```python
from build123d import *

# Parameters (mm, degrees)
SKETCH1_W               = 50
SKETCH1_H               = 50
SKETCH1_R               = 3.75
SKETCH1_R_2             = 2.75
BOSS_EXTRUDE1_DEPTH     = 3
BOSS_EXTRUDE2_DEPTH     = 50
CUT_EXTRUDE2_DEPTH      = 2
SKETCH10_W              = 50
SKETCH10_H              = 2.047418662
BOSS_EXTRUDE6_DEPTH     = 2
SKETCH11_W              = 5
SKETCH11_H              = 19
CUT_EXTRUDE4_DEPTH      = 4
SKETCH12_W              = 2
SKETCH12_H              = 50
BOSS_EXTRUDE7_DEPTH     = 10
SKETCH13_W              = 19
SKETCH13_H              = 5
CUT_EXTRUDE5_DEPTH      = 10
SKETCH14_R              = 5.75
SKETCH14_R_2            = 3.75
SKETCH14_R_3            = 4.75
SKETCH14_R_4            = 2.75
BOSS_EXTRUDE8_DEPTH     = 5
SKETCH15_W              = 50
SKETCH15_H              = 3
CUT_EXTRUDE6_DEPTH      = 161
CUT_EXTRUDE6_DEPTH_BACK = 15
SKETCH16_R              = 3.75
SKETCH16_R_2            = 2.75
BOSS_EXTRUDE9_DEPTH     = 8
SKETCH17_R              = 3.75
CUT_EXTRUDE7_DEPTH      = 9
SKETCH18_R              = 6
SKETCH18_R_2            = 4.75
BOSS_EXTRUDE10_DEPTH    = 8


with BuildPart() as part:
    # Sketch1 → Boss-Extrude1 (new body)
    with BuildSketch(Plane(origin=(0, 0, 0), x_dir=(1, 0, 0), z_dir=(0, 1, 0))):
        with Locations((0, 8.75)):
            Rectangle(SKETCH1_W, SKETCH1_H)
        Circle(SKETCH1_R, mode=Mode.SUBTRACT)
        with Locations((0, 17.5)):
            Circle(SKETCH1_R_2, mode=Mode.SUBTRACT)
    extrude(amount=BOSS_EXTRUDE1_DEPTH)

    # Sketch2 → Boss-Extrude2 (add)
    with BuildSketch(Plane.XY.offset(16.25)):
        Polygon((-25, 0), (-26.278653628, 0), (-74.233131713, 49.952581338), (-85, 49.952581338), (-85, 52), (-75, 52), (-75, 62), (-73, 62), (-73, 53), (-25, 3), align=None)
    boss_extrude2 = extrude(amount=-BOSS_EXTRUDE2_DEPTH)

    # Sketch3 → Cut-Extrude2 (cut)
    with BuildSketch(Plane(origin=(-11.511240633, -11.050791007, 0), x_dir=(0, 0, -1), z_dir=(0.721387321, 0.692531828, 0))):
        Polygon((-13.25, 85.788351472), (30.75, 85.788351472), (8.75, 25.788351472), align=None)
        Polygon((30.75, 77.073872213), (11.75, 25.255690395), (11.75, 19.477457668), (30.75, 19.477457668), (30.75, 22.897932802), align=None)
        Polygon((-13.25, 77.073872213), (-13.25, 19.477457668), (5.75, 19.477457668), (5.75, 25.255690395), align=None)
    cut_extrude2 = extrude(amount=-CUT_EXTRUDE2_DEPTH, mode=Mode.SUBTRACT)

    # Mirror1: Boss-Extrude2, Cut-Extrude2 across plane
    add(boss_extrude2.mirror(Plane(origin=(0, 0, 0), x_dir=(0, 0, 1), z_dir=(1, 0, 0))))
    add(cut_extrude2.mirror(Plane(origin=(0, 0, 0), x_dir=(0, 0, 1), z_dir=(1, 0, 0))), mode=Mode.SUBTRACT)

    # Sketch10 → Boss-Extrude6 (add)
    with BuildSketch(Plane(origin=(85, 0, 0), x_dir=(0, 0, -1), z_dir=(1, 0, 0))):
        with Locations((8.75, 50.976290669)):
            Rectangle(SKETCH10_W, SKETCH10_H)
    boss_extrude6 = extrude(amount=BOSS_EXTRUDE6_DEPTH)

    # Sketch11 → Cut-Extrude4 (cut)
    with BuildSketch(Plane(origin=(0, 49.952581338, 0), x_dir=(-1, 0, 0), z_dir=(0, -1, 0))):
        with Locations((-81.5, -3.75)):
            Rectangle(SKETCH11_W, SKETCH11_H)
        with Locations((-81.5, 21.25)):
            Rectangle(SKETCH11_W, SKETCH11_H)
    cut_extrude4 = extrude(amount=-CUT_EXTRUDE4_DEPTH, mode=Mode.SUBTRACT)

    # Mirror2: Boss-Extrude6, Cut-Extrude4 across plane
    add(boss_extrude6.mirror(Plane(origin=(0, 0, 0), x_dir=(0, 0, 1), z_dir=(1, 0, 0))))
    add(cut_extrude4.mirror(Plane(origin=(0, 0, 0), x_dir=(0, 0, 1), z_dir=(1, 0, 0))), mode=Mode.SUBTRACT)

    # Sketch12 → Boss-Extrude7 (add)
    with BuildSketch(Plane(origin=(0, 62, 0), x_dir=(1, 0, 0), z_dir=(0, 1, 0))):
        with Locations((74, 8.75)):
            Rectangle(SKETCH12_W, SKETCH12_H)
        with Locations((-74, 8.75)):
            Rectangle(SKETCH12_W, SKETCH12_H)
    extrude(amount=BOSS_EXTRUDE7_DEPTH)

    # Sketch13 → Cut-Extrude5 (cut)
    with BuildSketch(Plane.ZY.offset(-73)):
        with Locations((-21.25, 62.5)):
            Rectangle(SKETCH13_W, SKETCH13_H)
        with Locations((3.75, 62.5)):
            Rectangle(SKETCH13_W, SKETCH13_H)
    cut_extrude5 = extrude(amount=-CUT_EXTRUDE5_DEPTH, mode=Mode.SUBTRACT)

    # Mirror3: Cut-Extrude5 across plane
    add(cut_extrude5.mirror(Plane(origin=(0, 0, 0), x_dir=(0, 0, 1), z_dir=(1, 0, 0))), mode=Mode.SUBTRACT)

    # Sketch14 → Boss-Extrude8 (add)
    with BuildSketch(Plane(origin=(0, 3, 0), x_dir=(1, 0, 0), z_dir=(0, 1, 0))):
        Circle(SKETCH14_R)
        Circle(SKETCH14_R_2, mode=Mode.SUBTRACT)
        with Locations((0, 17.5)):
            Circle(SKETCH14_R_3)
        with Locations((0, 17.5)):
            Circle(SKETCH14_R_4, mode=Mode.SUBTRACT)
    extrude(amount=BOSS_EXTRUDE8_DEPTH)

    # Sketch15 → Cut-Extrude6 (cut, two sides)
    with BuildSketch(Plane.ZY.offset(-73)) as cut_extrude6_sk:
        with Locations((-8.75, 70.5)):
            Rectangle(SKETCH15_W, SKETCH15_H)
    extrude(amount=CUT_EXTRUDE6_DEPTH, mode=Mode.SUBTRACT)
    extrude(cut_extrude6_sk.sketch, amount=-CUT_EXTRUDE6_DEPTH_BACK, mode=Mode.SUBTRACT)

    # Sketch16 → Boss-Extrude9 (add)
    with BuildSketch(Plane(origin=(0, 8, 0), x_dir=(1, 0, 0), z_dir=(0, 1, 0))):
        Circle(SKETCH16_R)
        Circle(SKETCH16_R_2, mode=Mode.SUBTRACT)
    extrude(amount=-BOSS_EXTRUDE9_DEPTH)

    # Sketch17 → Cut-Extrude7 (cut, through all)
    with BuildSketch(Plane(origin=(0, 8, 0), x_dir=(1, 0, 0), z_dir=(0, 1, 0))):
        with Locations((0, 17.5)):
            Circle(SKETCH17_R)
    extrude(amount=-CUT_EXTRUDE7_DEPTH, mode=Mode.SUBTRACT)

    # Sketch18 → Boss-Extrude10 (add)
    with BuildSketch(Plane(origin=(0, 8, 0), x_dir=(1, 0, 0), z_dir=(0, 1, 0))):
        with Locations((0, 17.5)):
            Circle(SKETCH18_R)
        with Locations((0, 17.5)):
            Circle(SKETCH18_R_2, mode=Mode.SUBTRACT)
    extrude(amount=-BOSS_EXTRUDE10_DEPTH)


solid = part.part
```
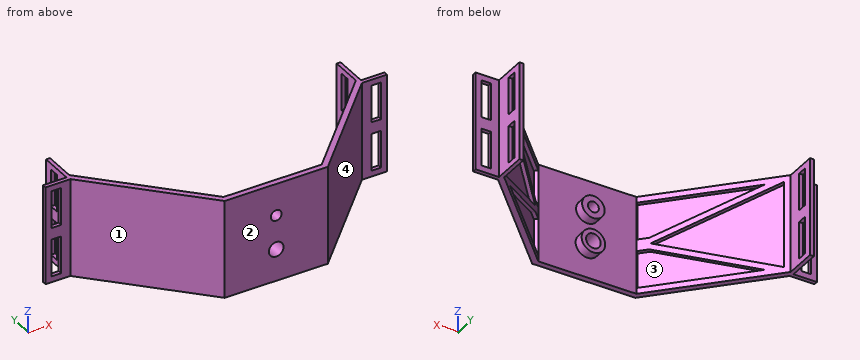
Model file for the job. Use its own axes, mm. Face numbers are marked on the shaded views. Give positions to 0.01 mm unless a question says otherwise; leave off trailing zeros. Loops run counter-clockwise (first coordinate to the right, second up) from the corner with the lowest first, then second, coordinate; pieces in that order, holes last. Notation, with made-up numbers: (-33, -17.75) -> (19, -17.75) arc R15 cw to (19, 9.25) -> close; hole circle Ø7 at (-24, -12). An arc over 180 degrees is marked (long way). Write each question's results on one line, items separated by ' | '.
(1) Flat gauge pins, fed straight in: pin 1 Ø5 at (x, z) = (-66.5, 3) entering from -Y; pin 2 Ø12 at (x, z) = (49.5, -9) entering from -Y; pin 3 Ø20.5 at (x, y) = (47, 27.5) entering from -Z; pin 4 Ø2 at (x, z) = (25.5, -19.5) entering from +Y. Where does each tip first touch, or does it go through?
Geometry results:
pin 1: stops at y = 39.29 | pin 2: stops at y = 17.94 | pin 3: stops at z = -33.75 | pin 4: stops at y = 3
(2) Cut at D-D on x = 20.5. List the corners of the cut face in (y, z).
Geometry results:
outline: (0, -33.75) -> (3, -33.75) -> (3, 16.25) -> (0, 16.25) -> close
(3) Probe line 1 along Z through (x, y) = (0, 3.75); line 2 along Z through (x, y) = (0, 2); line 3 along X through (y, z) = (54.5, 11.5). List the from-to ranges inside material, lowest first.
Geometry results:
line 1: z = -23.5 to -21.25, -13.75 to -11.5, -5.75 to -2.75, 2.75 to 5.75 | line 2: z = -33.75 to -21.25, -13.75 to -2.75, 2.75 to 16.25 | line 3: x = -75 to -73, 73 to 75
(4) Cut at A-A on x = 0. List the corners of the cut face in (y, z).
Geometry results:
outline: (0, -33.75) -> (3, -33.75) -> (3, -23.5) -> (8, -23.5) -> (8, -21.25) -> (0, -21.25) -> close; (0, -13.75) -> (8, -13.75) -> (8, -11.5) -> (3, -11.5) -> (3, -5.75) -> (8, -5.75) -> (8, -2.75) -> (0, -2.75) -> close; (0, 2.75) -> (8, 2.75) -> (8, 5.75) -> (3, 5.75) -> (3, 16.25) -> (0, 16.25) -> close
(5) Pull direction X, two halves, no side cores. Call the marked faces 1, 2, 3 and 4: released by +X, released by -X, zero draft, split by the parting line, or undercut.
Geometry results:
face 1: released by -X | face 2: zero draft | face 3: undercut | face 4: released by +X
(6) Cut at C-C on y = 63. List the corners of the cut face in (x, z), and give its area (3 significant figures).
Geometry results:
outline: (-75, -33.75) -> (-73, -33.75) -> (-73, -30.75) -> (-75, -30.75) -> close; (-75, -11.75) -> (-73, -11.75) -> (-73, -5.75) -> (-75, -5.75) -> close; (-75, 13.25) -> (-73, 13.25) -> (-73, 16.25) -> (-75, 16.25) -> close; (73, -33.75) -> (75, -33.75) -> (75, -30.75) -> (73, -30.75) -> close; (73, -11.75) -> (75, -11.75) -> (75, -5.75) -> (73, -5.75) -> close; (73, 13.25) -> (75, 13.25) -> (75, 16.25) -> (73, 16.25) -> close | area: 48.0 mm²
